Could you check a few things on this model? Use its own coordinates, in mm. Face numbers are marked on the shaded views. A direction names the side the tool comes from. Coordinates: 2 decimals unless noted, no trailing zeros. Loops run counter-clockwise (first coordinate to the right, second up) from the corner with the lowest first, then second, coordinate; pieces in that order, holes last.
from build123d import *

# Parameters (mm, degrees)
SKETCH3_W          = 4.7752
SKETCH3_H          = 4.7752
CUT_EXTRUDE1_DEPTH = 92.298779839


with BuildPart() as part:
    # Sketch1 → Revolve1 (revolve)
    with BuildSketch(Plane.XY, mode=Mode.PRIVATE) as revolve1_sk:
        with BuildLine():
            Line((-38.1, 35.56), (-19.05, 35.56))
            Line((-19.05, 35.56), (-19.05, 31.75))
            Line((-19.05, 31.75), (0, 31.75))
            Line((0, 31.75), (0, 28.448))
            Line((0, 28.448), (19.05, 28.448))
            Line((19.05, 28.448), (19.05, 25.4))
            Line((19.05, 25.4), (38.1, 25.4))
            Line((38.1, 25.4), (38.1, 12.7))
            Line((38.1, 12.7), (-6.61235224, 12.7))
            ThreePointArc((-6.61235224, 12.7), (-10.239814738, 21.587016556), (-19.05, 25.39728992))
            Line((-19.05, 25.39728992), (-19.096408435, 25.4))
            Line((-19.096408435, 25.4), (-38.1, 25.4))
            Line((-38.1, 25.4), (-38.1, 35.56))
        make_face()
    revolve(revolve1_sk.sketch.rotate(Axis((-38.1, 0, 0), (1, 0, 0)), 90), axis=Axis((-38.1, 0, 0), (1, 0, 0)))

    # Sketch3 → Cut-Extrude1 (cut, through all)
    with BuildSketch(Plane(origin=(38.1, 0, 0), x_dir=(0, 0, -1), z_dir=(1, 0, 0))):
        with Locations((12.7, 0)):
            Rectangle(SKETCH3_W, SKETCH3_H)
    extrude(amount=-CUT_EXTRUDE1_DEPTH, mode=Mode.SUBTRACT)


solid = part.part
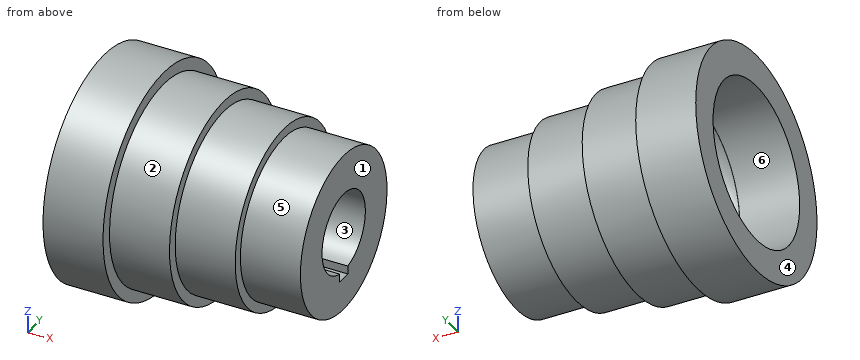
1) If I drill on L1, parallel to Y at x = 27, z = 0; L2, parallel to Y at x = 10, z = 0; L3, parallel to Z at x = 14.5, y = 3, over which ranges is the centre line in solid material (lowest first)?
2) Imagine slicing it at A-A on x = 15. List the corners of the cut face in (y, z) for me.
3) Imagine slicing it at C-C on x = -26.5. List the corners of the cut face in (y, z) for me.
4) Will these pins go through, and if not, where does the flat tip stop? pin 1 (1.3 mm diameter, centred on x = 22.5, z = -14, fed in from -Y); pin 2 (3 mm diameter, centred on x = 20, z = -24.5, fed in from -Y); pin 3 (6 mm diameter, centred on y = -19, z = -2, fed in from -X); pin 4 (15 mm diameter, centred on y = 0, z = 0, fed in from -X).
5) Imagine slicing it at B-B on y = -30. List the corners of the cut face in (x, z) for me.
6) For the marked faces 4, 5 and 6, which set-ups out of +Z, -Z, +X, -X, +Y, -Y let a thin tool reach every point of the face, with its end or its side?
7) We'd pull the mould along Z, two halves only. Please class the marked faces 1, 2 and 3: released by +Z, released by -Z, zero draft, split by the parting line, or undercut.
Solved:
1. L1: y = -25.4 to -12.7, 12.7 to 25.4
1. L2: y = -28.45 to -12.7, 12.7 to 28.45
1. L3: z = -28.29 to -12.34, 12.34 to 28.29
2. outline: circle Ø56.9 at (0, 0); hole (-2.39, -15.09) - (2.39, -15.09) - (2.39, -12.47) arc R12.7 ccw (long way) to (-2.39, -12.47) - close
3. outline: circle Ø71.12 at (0, 0); hole circle Ø50.8 at (0, 0)
4. pin 1: stops at y = -21.61
4. pin 2: stops at y = -16.27
4. pin 3: stops at x = -10.78
4. pin 4: passes through
5. outline: (-38.1, -19.09) - (-19.05, -19.09) - (-19.05, -10.4) - (0, -10.4) - (0, 10.4) - (-19.05, 10.4) - (-19.05, 19.09) - (-38.1, 19.09) - close
6. face 4: +Z, -Z, -X, +Y, -Y
6. face 5: +X
6. face 6: -X
7. face 1: zero draft
7. face 2: split by the parting line
7. face 3: undercut
